Part print with two shaded views. Sizes in mm from the minimum x, y, z corner. A direction names the side the tool comes from. Give positions to 0.01 mm unless a question says otherwise; leave off trailing zeros. Write each loop counter-clockwise with the first axis right and the second up, starting at its lowest first coordinate (ties: lowest second). Pieces come first, ordered by that corner, then holes. Notation, with made-up numbers: (69, 28.25) -> (102, 28.25) arc R11 cw to (102, 36.25) -> close; hole circle Ø6 at (20, 11). An arc over 180 degrees is marked (long way). Answer as a JSON object with one key per item and string values.
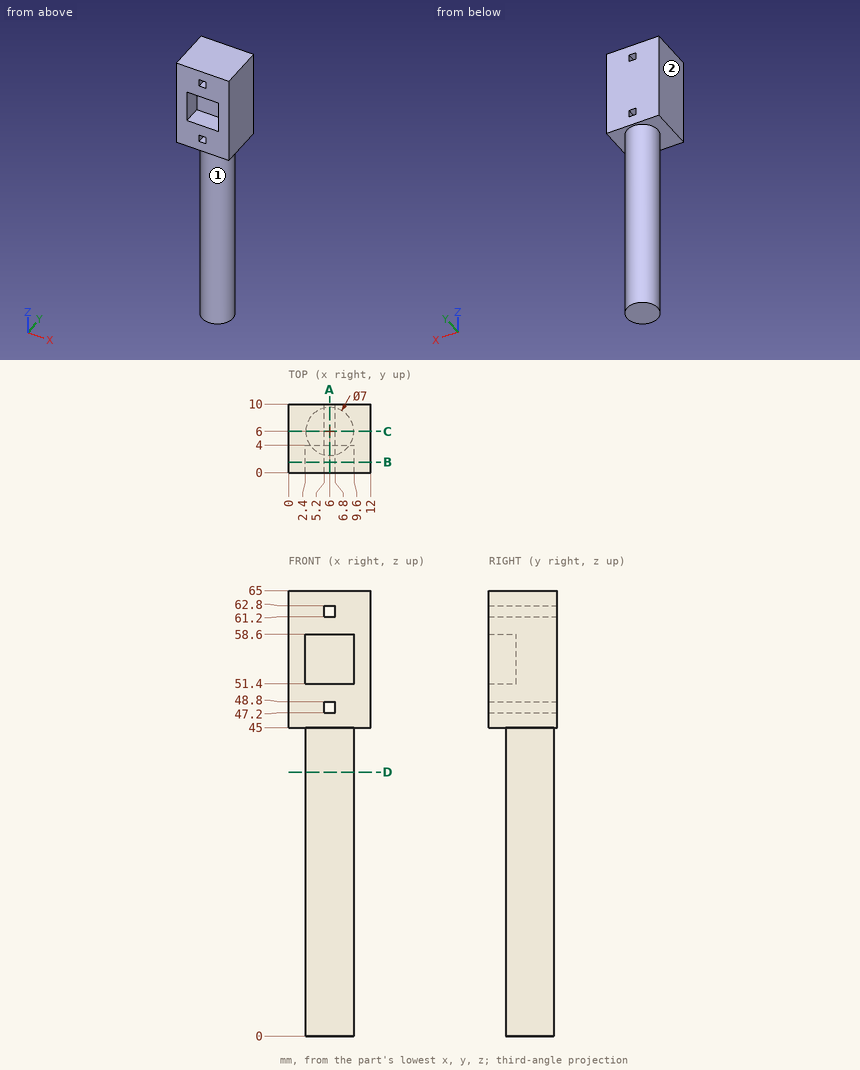
1) Slice it at C-C (y = 6). List the corners of the cut face in (x, z), then the cut area to 3 significant figures.
Model answer:
{"outline": "(0, 45) -> (2.5, 45) -> (2.5, 0) -> (9.5, 0) -> (9.5, 45) -> (12, 45) -> (12, 65) -> (0, 65) -> close; hole (5.2, 47.2) -> (6.8, 47.2) -> (6.8, 48.8) -> (5.2, 48.8) -> close; hole (5.2, 61.2) -> (6.8, 61.2) -> (6.8, 62.8) -> (5.2, 62.8) -> close", "area": "550 mm2"}
2) Pin check, flat tips, straight feed: pin 1 (6 mm diameter, centred on y = 1.5, z = 18, fed in from +X); pin 2 (4 mm diameter, centred on y = 3, z = 41, fed in from +X); pin 3 (5 mm diameter, centred on x = 7, z = 10.5, fed in from -Y). Stop position of each tip, or through.
Model answer:
{"pin 1": "stops at x = 9.16", "pin 2": "stops at x = 9.35", "pin 3": "stops at y = 2.5"}
3) Wall check: probe 1 along Z at (x, y) = (5.25, 3.75); probe 2 along X at (y, z) = (3, 55); probe 3 along X at (y, z) = (1.75, 61.5). Give the ranges that are in metal, low to high.
Model answer:
{"probe 1": "z = 0 to 47.2, 48.8 to 51.4, 58.6 to 61.2, 62.8 to 65", "probe 2": "x = 0 to 2.4, 9.6 to 12", "probe 3": "x = 0 to 5.2, 6.8 to 12"}
4) Slice it at B-B (y = 1.5). List the corners of the cut face in (x, z), then the cut area to 3 significant figures.
Model answer:
{"outline": "(0, 45) -> (12, 45) -> (12, 65) -> (0, 65) -> close; hole (2.4, 51.4) -> (9.6, 51.4) -> (9.6, 58.6) -> (2.4, 58.6) -> close; hole (5.2, 47.2) -> (6.8, 47.2) -> (6.8, 48.8) -> (5.2, 48.8) -> close; hole (5.2, 61.2) -> (6.8, 61.2) -> (6.8, 62.8) -> (5.2, 62.8) -> close", "area": "183 mm2"}
5) Slice it at D-D (z = 38.5). List the corners of the cut face in (x, y).
Model answer:
{"outline": "circle Ø7 at (6, 6)"}
6) 3-axis set-ups, long thin cutter, end or side, ignore diameter. For the marked faces 1 and 2: which of +Z, -Z, +X, -X, +Y, -Y reach the whole face in a straight line?
Model answer:
{"face 1": "-Z", "face 2": "+Z, -Z, -X, +Y, -Y"}
7) Slice it at A-A (x = 6). List the corners of the cut face in (y, z), then the cut area to 3 significant figures.
Model answer:
{"outline": "(0, 45) -> (2.5, 45) -> (2.5, 0) -> (9.5, 0) -> (9.5, 45) -> (10, 45) -> (10, 47.2) -> (0, 47.2) -> close; (0, 48.8) -> (10, 48.8) -> (10, 61.2) -> (0, 61.2) -> (0, 58.6) -> (4, 58.6) -> (4, 51.4) -> (0, 51.4) -> close; (0, 62.8) -> (10, 62.8) -> (10, 65) -> (0, 65) -> close", "area": "454 mm2"}
